For this review, take the finished solid that the model builds, in its own axes (mm). Face numbers are marked on the shaded views. Coordinates: 2 decimals unless noted, no trailing zeros. Write each loop counter-clockwise with the first axis right and the second up, starting at its lowest first coordinate (ties: lowest second). Pieces come first, ordered by that corner, then holes.
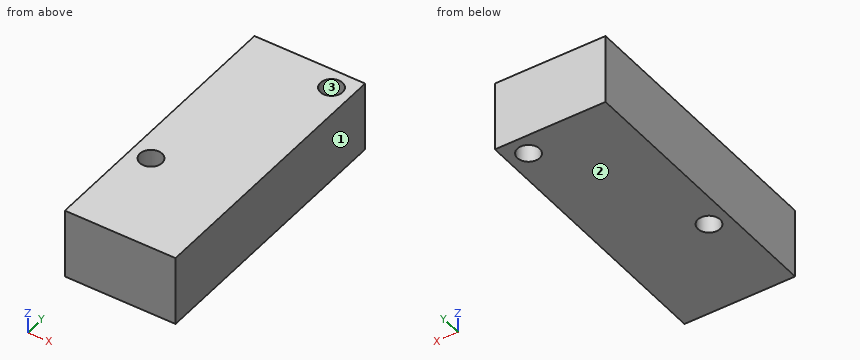
Autodesk Inventor part; units mm, degrees
ref_plane "YZ Plane" through (0, 0, 0) normal (1, 0, 0) x (0, 1, 0)
ref_plane "XZ Plane" through (0, 0, 0) normal (0, 1, 0) x (-1, 0, 0)
ref_plane "XY Plane" through (0, 0, 0) normal (0, 0, 1) x (1, 0, 0)
sketch "Sketch1" plane through (0, 0, 0) normal (0, 0, 1) x (1, 0, 0)
  line L0 (0, 0) -> (0, 28.7274)
  line L1 (0, 28.7274) -> (15.8242, 28.7274)
  line L2 (15.8242, 28.7274) -> (15.8242, 0)
  line L3 (15.8242, 0) -> (0, 0)
  circle A0 centre (12.9667, 25.8699) radius 1.5875
  circle A1 centre (12.9667, 25.8699) radius 2.8575
  circle A2 centre (2.8575, 2.8575) radius 1.5875
  circle A3 centre (2.8575, 2.8575) radius 2.8575
  dimension "d0" = 28.7274
  dimension "d1" = 15.8242
  dimension "d2" = 3.175
  dimension "d3" = 5.715
  dimension "d4" = 3.175
  dimension "d5" = 5.715
extrude "Extrusion1" add sketch "Sketch1" along normal blind 10.0076
sketch "Sketch2" plane through (0, 0, 10.0076) normal (0, 0, 1) x (1, 0, 0)
  line L0 (0, 0) -> (15.8242, 0)
  line L1 (15.8242, 28.7274) -> (0, 28.7274)
  line L2 (0, 0) -> (0, -10.9982)
  line L3 (0, -10.9982) -> (15.8242, -10.9982)
  line L4 (15.8242, -10.9982) -> (15.8242, 0)
  dimension "d8" = 10.9982
extrude "Extrusion2" add sketch "Sketch2" against normal blind 10.0076
properties part number "Limit Switch"
Q1. Add section C-C (z = 1). State the section outline as (x, y) points (1 decimal), then the cut area to 3 significant figures.
Ans:
outline: (0, -11) - (15.8, -11) - (15.8, 28.7) - (0, 28.7) - close; hole circle Ø3.2 at (2.9, 2.9); hole circle Ø3.2 at (13, 25.9)
area: 613 mm2
Q2. Draft analysis for pull direction X (two halves, no side actions). For the marked faces 1, 2 and 3, state which applies: +X half, -X half, draft (parallel to the pull), parting line (faces both ways), or undercut.
Ans:
face 1: +X half
face 2: draft
face 3: undercut
Q3. Add section B-B (x = 13). State the section outline as (y, z) points, then the cut area to 3 significant figures.
Ans:
outline: (-11, 0) - (24.28, 0) - (24.28, 10.01) - (-11, 10.01) - close; (27.46, 0) - (28.73, 0) - (28.73, 10.01) - (27.46, 10.01) - close
area: 366 mm2
Q4. For probe 1 along Y at (x, z) = (12, 6.5); probe 2 along Y at (x, z) = (13.75, 8.25); probe 3 along X at (y, z) = (4, 8.25), list the stretches that pass through material, from the lowest coordinate up.
Ans:
probe 1: y = -11 to 24.61, 27.13 to 28.73
probe 2: y = -11 to 24.49, 27.25 to 28.73
probe 3: x = 0 to 1.76, 3.96 to 15.82
Q5. Add section A-A (y = 3.5). State the section outline as (x, z) points, then the cut area to 3 significant figures.
Ans:
outline: (0, 0) - (1.41, 0) - (1.41, 10.01) - (0, 10.01) - close; (4.31, 0) - (15.82, 0) - (15.82, 10.01) - (4.31, 10.01) - close
area: 129 mm2
Q6. Clearance check with a flat-ended pin moving along its axis: pin 1 Ø2.5 at (x, y) = (2.86, 2.86) entering from -Z. State where the tip first meets the part, or that it passes through.
Ans:
pin 1: passes through
